Could you check a few things on this model? Use its own coordinates, in mm. Face numbers are marked on the shaded views. A direction names the side the tool comes from. Round coordinates to 2 decimals unless told otherwise and drop trailing zeros. Order: outer loops, then holes, each group sorted by start corner. A loop starts at its lowest first (then second) coordinate and runs counter-clockwise, first axis right, second up. Notation, with made-up numbers: (47.5, -15) -> (80.5, -15) arc R7 ccw to (80.5, -11) -> close; hole circle Ø5 at (25, 88.25). An arc over 180 degrees is marked (long way). Put each result on its own line as item: value. Start each with the question number.
from build123d import *

# Parameters (mm, degrees)
F_3_5_3_5_DIAMETER_HOLE1_AT_2_COUNT = 2
F_3_5_3_5_DIAMETER_HOLE1_AT_2_PITCH = 11.313708499
F_3_5_3_5_DIAMETER_HOLE1_AT_3_COUNT = 2
F_3_5_3_5_DIAMETER_HOLE1_AT_3_PITCH = 16
F_3_5_3_5_DIAMETER_HOLE1_AT_4_COUNT = 2
F_3_5_3_5_DIAMETER_HOLE1_AT_4_PITCH = 11.313708499
CHAMFER1_SIZE                       = 0.25


with BuildPart() as part:
    # Sketch1 → Revolve1 (revolve)
    with BuildSketch(Plane.XY, mode=Mode.PRIVATE) as revolve1_sk:
        Polygon((7.525, 0), (7.525, 5.035), (-2.575, 5.035), (-2.575, 11), (-6.025, 11), (-6.025, 5.035), (-7.525, 5.035), (-7.525, 0), align=None)
    revolve(revolve1_sk.sketch.rotate(Axis((-7.525, 0, 0), (1, 0, 0)), 90), axis=Axis((-7.525, 0, 0), (1, 0, 0)))

    # Sketch3 → Ø8.0 (8) Diameter Hole1 (revolve, cut)
    with BuildSketch(Plane(origin=(-7.525, 0, 0), x_dir=(0, 0, 1), z_dir=(0, 1, 0))):
        Polygon((0, 0), (0, 15.05), (4.25, 15.05), (4, 14.8), (4, 0.25), (4.25, 0), align=None)
    revolve(axis=Axis((-13.875, 0, 0), (1, 0, 0)), mode=Mode.SUBTRACT)

    # Sketch7 → Ø3.5 (3.5) Diameter Hole1 (revolve, cut)
    with BuildSketch(Plane(origin=(-6.025, 8, 0), x_dir=(0, 0, 1), z_dir=(0, 1, 0))):
        Polygon((0, 0), (0, 3.45), (1.8, 3.45), (1.75, 3.4), (1.75, 0.05), (1.8, 0), align=None)
    f_3_5_3_5_diameter_hole1 = revolve(axis=Axis((-12.375, 8, 0), (1, 0, 0)), mode=Mode.SUBTRACT)

    # Ø3.5 (3.5) Diameter Hole1 at 2: Ø3.5 (3.5) Diameter Hole1 ×2
    with Locations(*[Vector(0, -0.7071067811865476, 0.7071067811865476) * (i * F_3_5_3_5_DIAMETER_HOLE1_AT_2_PITCH) for i in range(1, F_3_5_3_5_DIAMETER_HOLE1_AT_2_COUNT)]):
        add(f_3_5_3_5_diameter_hole1, mode=Mode.SUBTRACT)

    # Ø3.5 (3.5) Diameter Hole1 at 3: Ø3.5 (3.5) Diameter Hole1 ×2
    with Locations(*[(0, -i * F_3_5_3_5_DIAMETER_HOLE1_AT_3_PITCH, 0) for i in range(1, F_3_5_3_5_DIAMETER_HOLE1_AT_3_COUNT)]):
        add(f_3_5_3_5_diameter_hole1, mode=Mode.SUBTRACT)

    # Ø3.5 (3.5) Diameter Hole1 at 4: Ø3.5 (3.5) Diameter Hole1 ×2
    with Locations(*[Vector(0, -0.7071067811865476, -0.7071067811865476) * (i * F_3_5_3_5_DIAMETER_HOLE1_AT_4_PITCH) for i in range(1, F_3_5_3_5_DIAMETER_HOLE1_AT_4_COUNT)]):
        add(f_3_5_3_5_diameter_hole1, mode=Mode.SUBTRACT)

    # Chamfer1
    chamfer1_edges = [part.edges().sort_by_distance(p)[0] for p in [
        (-6.025, 0, -11),
        (-2.575, 0, -11),
    ]]
    chamfer(chamfer1_edges, length=CHAMFER1_SIZE)


solid = part.part
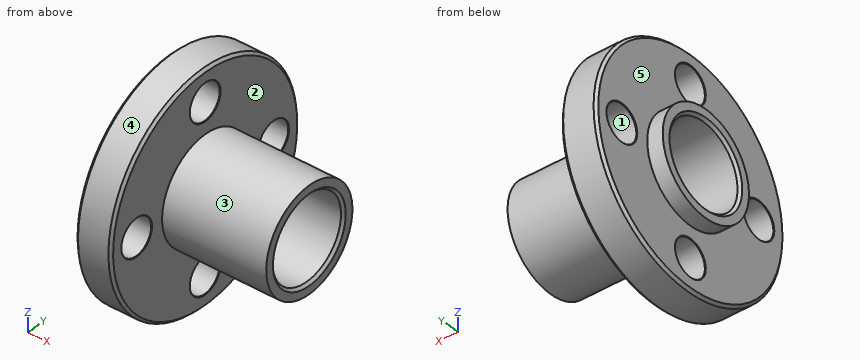
1. For pin 1 Ø6.5 at (y, z) = (0, 0) entering from -X; pin 2 Ø2 at (y, z) = (8.5, -7.5) entering from +X (3 decimals); pin 3 Ø12 at (y, z) = (1.5, -0.5) entering from +X (3 decimals); pin 4 Ø4 at (x, z) = (1, 3) entering from +Y, each with a flat end and sliding along its axis, tell me the tip position at first contact or that it passes through.
2. If we section it at B-B, the plane z = 0: Count the separate pieces of the cut face and the enclosed holes in it, then the cut area to 3 significant figures.
3. Which directions (+Z, -Z, +X, -X, +Y, -Y) give clear straight access to the entire face, cutting with the end or side of a thin tool? Please do the marked faces 4 and 5.
4. If we section it at A-A, the plane x = -0.5: Please give me the cut outline in (y, z) (3 decimals), then the cut area to 3 significant figures.
5. Thinking about a two-plate mould opening in Y: for the marked faces 1, 2 and 3, which applies, +Y half, -Y half, draft (parallel to the pull), parting line (faces both ways), or undercut?
6. I need wall thicknesses on L1, parallel to Y at x = -0.5, z = 0 (3 decimals); L2, parallel to X at y = 7.75, z = 5.5 (3 decimals); L3, parallel to Y at x = -2.5, z = 3.5. Which ranges of each line are inside material? Lowest first, please.
Results below:
1. pin 1: through
1. pin 2: x = -2.575
1. pin 3: x = 7.525
1. pin 4: y = 4.93
2. separate pieces: 4
2. enclosed holes: 0
2. area: 47.9 mm2
3. face 4: +X, -X
3. face 5: -X
4. outline: circle Ø10.07 at (0, 0); hole circle Ø8 at (0, 0)
4. area: 29.4 mm2
5. face 1: undercut
5. face 2: draft
5. face 3: parting line
6. L1: -5.035 to -4, 4 to 5.035
6. L2: -6.025 to -2.575
6. L3: -3.62 to -1.94, 1.94 to 3.62
